Geometry: final body of the model. Coordinates: model frame, mm. Face numbers are marked on the shaded views. A direction names the side the tool comes from. Coordinates: 2 decimals unless noted, no trailing zeros. Write each loop counter-clockwise with the first axis right and the second up, starting at its lowest first coordinate (ties: lowest second). Pieces come first, ordered by that corner, then holes.
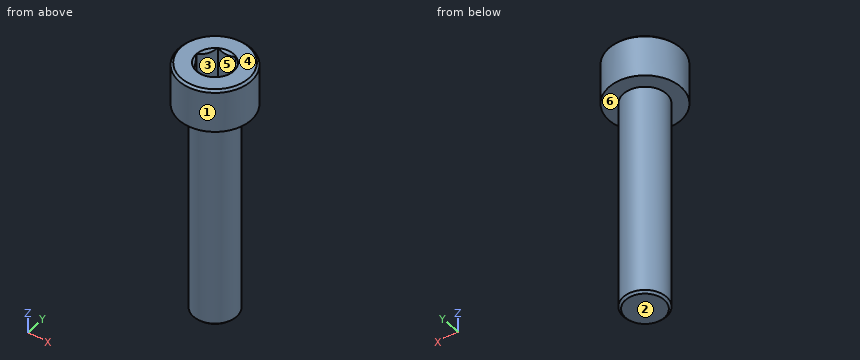
from build123d import *

# Parameters (mm, degrees)
SKETCH_1_R          = 3.35
EXTRUDE_1_DEPTH     = 4
CUT_EXTRUDE_1_DEPTH = 2.8
SKETCH_3_R          = 2
EXTRUDE_2_DEPTH     = 20
SKETCH_4_R          = 1.732050808
CUT_EXTRUDE_2_DEPTH = 2
CUT_EXTRUDE_2_DRAFT = -45
CHAMFER_1_SIZE      = 0.2


with BuildPart() as part:
    # Эскиз1 → Бобышка-Вытянуть1 (new body)
    with BuildSketch(Plane.XY):
        Circle(SKETCH_1_R)
    extrude(amount=EXTRUDE_1_DEPTH)

    # Эскиз2 → Вырез-Вытянуть1 (cut)
    with BuildSketch(Plane.XY.offset(4)):
        Polygon((1.732050808, 0), (0.866025404, 1.5), (-0.866025404, 1.5), (-1.732050808, 0), (-0.866025404, -1.5), (0.866025404, -1.5), align=None)
    extrude(amount=-CUT_EXTRUDE_1_DEPTH, mode=Mode.SUBTRACT)

    # Эскиз3 → Бобышка-Вытянуть2 (add)
    with BuildSketch(Plane(origin=(0, 0, 0), x_dir=(-1, 0, 0), z_dir=(0, 0, -1))):
        Circle(SKETCH_3_R)
    extrude(amount=EXTRUDE_2_DEPTH)


with BuildPart() as cut_extrude_2_tool:
    # Эскиз4 → Вырез-Вытянуть2 (with draft: the straight prism first)
    with BuildSketch(Plane.XY.offset(4)):
        Circle(SKETCH_4_R)
    extrude(amount=-CUT_EXTRUDE_2_DEPTH)
    # Вырез-Вытянуть2: the draft: its side faces are tilted about the plane it starts from
    cut_extrude_2_sides = [cut_extrude_2_tool.faces().sort_by_distance(p)[0] for p in [
        (-1.732050808, 0, 3),
    ]]
    draft(cut_extrude_2_sides, Plane.XY.offset(4), CUT_EXTRUDE_2_DRAFT)


with BuildPart() as part_1:
    add(part.part)

    # Вырез-Вытянуть2: cut by cut_extrude_2_tool
    add(cut_extrude_2_tool.part, mode=Mode.SUBTRACT)

    # Фаска1
    chamfer_1_edges = [part_1.edges().sort_by_distance(p)[0] for p in [
        (2, 0, -20),
        (-3.35, 0, 4),
    ]]
    chamfer(chamfer_1_edges, length=CHAMFER_1_SIZE)


solid = part_1.part
Item 1: Pull-direction query (Y, two-part tool) for the marked faces 1, 2 and 3; classes: released by +Y, released by -Y, zero draft, split by the parting line, or undercut.
Derived:
face 1: split by the parting line
face 2: zero draft
face 3: undercut
Item 2: Section A-A, the plane x = 0. Output: boundary loops of the cut face in (y, z).
Derived:
outline: (-3.35, 0) - (-2, 0) - (-2, -19.8) - (-1.8, -20) - (1.8, -20) - (2, -19.8) - (2, 0) - (3.35, 0) - (3.35, 3.8) - (3.15, 4) - (1.73, 4) - (1.5, 3.77) - (1.5, 1.2) - (-1.5, 1.2) - (-1.5, 3.77) - (-1.73, 4) - (-3.15, 4) - (-3.35, 3.8) - close
Item 3: Section B-B, the plane z = -17.75. Output: boundary loops of the cut face in (x, y).
Derived:
outline: circle Ø4 at (0, 0)
Item 4: Material intervals for probe 1 along Z at (x, y) = (-0.25, -2.5); probe 2 along X at (y, z) = (1, -16.25); probe 3 along Z at (x, y) = (-0.75, -0.75), sorted ascending.
Derived:
probe 1: z = 0 to 4
probe 2: x = -1.73 to 1.73
probe 3: z = -20 to 1.2
Item 5: Set-up query: the marked faces 4, 5 and 6. Return all of +Z, -Z, +X, -X, +Y, -Y with unobstructed straight access to the full face (end or side cutting, diameter ignored); none if empty.
Derived:
face 4: +Z, +X, -X, +Y, -Y
face 5: +Z
face 6: -Z
Item 6: Pin query (flat end, axial travel): pin 1 (2 mm diameter, centred on x = -1.5, z = -2, fed in from +Y); pin 2 (3 mm diameter, centred on y = -1.5, z = -17, fed in from -X); pin 3 (2 mm diameter, centred on x = 2, z = -13, fed in from -Y). Return the tip coordinate at first contact, or that it passes through.
Derived:
pin 1: stops at y = 1.94
pin 2: stops at x = -2
pin 3: stops at y = -1.73
